The listing builds one solid part. Answer for the finished solid, in the listing's coordinates (mm). A direction names the side the tool comes from. Coordinates: 2 decimals unless noted, no trailing zeros. Loops run counter-clockwise (first coordinate to the right, second up) from the corner with the lowest first, then second, coordinate; pieces in that order, holes last. Notation, with made-up numbers: (81.5, -32.5) - (88.5, -32.5) arc R24 cw to (88.5, -8.5) - close; hole circle Ø2 at (-34.75, 22). An arc over 180 degrees is marked (long way). Write each question's results on one line, items separated by ' | '. Start each with the question number.
(1) Find section C-C on y = 24.5. Determine the outline of the cut face in (x, z) (3 decimals), then the cut area to 3 significant figures.
(2) Determine the mould class of faces 1 (the flat face through (-41, 50.165, 7)), 2 (the flat face through (1, 32, -7.938)), 3 (the flat face through (1, 35.052, -2)) for opening direction Y: released by +Y, released by -Y, zero draft, split by the parting line, or undercut.
(3) Find section B-B on x = 16. Determine the outline of the cut face in (y, z).
(4) For faces 4 (the flat face through (1, -35.052, -2)), 5 (the flat face through (-31.75, 52, 7)), 6 (the flat face through (-1, 45, 3.549)), determine the directions among +Z, -Z, +X, -X, +Y, -Y from which every point of the face is accessible in a straight line to the end or side of a thin tool.
(5) Find section A-A on z = -2.5. Determine the outline of the cut face in (x, y).
(6) Given pin 1 Ø5.5 at (x, z) = (-8.5, -3) entering from +Y; pin 2 Ø3.5 at (x, z) = (21.5, -2) entering from -Y; pin 3 Ø3 at (x, y) = (20.5, 33) entering from +Z, each flat-ended and moving along its own axis, determine where each tip first touches the part or whether it passes through.
(7) Consider line 1 (Y direction, x = 19.5, z = -0.5); line 2 (Y direction, x = -3.5, z = 4.25); line 3 (X direction, y = -45, z = 7) (3 decimals). Determine where each line is inside the solid, lowest interval first. Write a range as from..to.
(8) Find section D-D on y = -43. Determine the outline of the cut face in (x, z) (3 decimals).
from build123d import *

# Parameters (mm, degrees)
F1_DEPTH      = 54.7751
F1_DEPTH_BACK = 54.7751
F3_DEPTH      = 54.7761
F3_DEPTH_BACK = 54.7761
F4_W          = 109.5502
F4_H          = 5.9763903179
F5_DEPTH      = 54.7751
F5_DEPTH_BACK = 54.7751
F7_DEPTH      = 4.4523903179
F8_W          = 57.404
F8_H          = 17.4625
F9_DEPTH      = 50.165
F9_DEPTH_BACK = 50.165
F10_W         = 1.27
F10_H         = 0.635
F10_W_2       = 0.635
F10_H_2       = 1.27
F11_DEPTH     = 4.4523903179


with BuildPart() as f1:
    # F0 (on Right) → F1 (new body, two sides)
    with BuildSketch(Plane.YZ) as f1_sk:
        Polygon((35.052, 9.525), (-35.052, 9.525), (-35.052, -7.9375), (-28.702, -7.9375), (-28.702, 0), (28.702, 0), (28.702, -7.9375), (35.052, -7.9375), align=None)
    extrude(amount=F1_DEPTH)
    extrude(f1_sk.sketch, amount=-F1_DEPTH_BACK)

    # F2 (on Right) → F3 (cut, two sides)
    with BuildSketch(Plane.YZ) as f3_sk:
        with BuildLine():
            ThreePointArc((28.702, 0), (0, 3.5486096821), (-28.702, 0))
            Line((-28.702, 0), (28.702, 0))
        make_face()
    extrude(amount=F3_DEPTH, mode=Mode.SUBTRACT)
    extrude(f3_sk.sketch, amount=-F3_DEPTH_BACK, mode=Mode.SUBTRACT)

    # F4 (on Right) → F5 (join, two sides)
    with BuildSketch(Plane.YZ) as f5_sk:
        with Locations((0, 6.536804841)):
            Rectangle(F4_W, F4_H)
    extrude(amount=F5_DEPTH)
    extrude(f5_sk.sketch, amount=-F5_DEPTH_BACK)

    # F6 (on face) → F7 (cut, through all)
    with BuildSketch(Plane.XY.offset(9.525)):
        Polygon((50.165, -50.165), (50.165, 50.165), (31.75, 50.165), (31.75, 54.7751), (-31.75, 54.7751), (-31.75, 50.165), (-50.165, 50.165), (-50.165, -50.165), (-31.75, -50.165), (-31.75, -54.7751), (31.75, -54.7751), (31.75, -50.165), align=None)
    extrude(amount=-F7_DEPTH, mode=Mode.SUBTRACT)

    # F8 (on Right) → F9 (cut, two sides)
    with BuildSketch(Plane.YZ) as f9_sk:
        with Locations((0, 0.79375)):
            Rectangle(F8_W, F8_H)
    extrude(amount=F9_DEPTH, mode=Mode.SUBTRACT)
    extrude(f9_sk.sketch, amount=-F9_DEPTH_BACK, mode=Mode.SUBTRACT)

    # F10 (on face) → F11 (join, through all)
    with BuildSketch(Plane.XY.offset(5.0726096821)):
        with Locations((-32.385, 49.8475)):
            Rectangle(F10_W, F10_H)
        with Locations((32.385, 49.8475)):
            Rectangle(F10_W, F10_H)
        with Locations((-32.385, -49.8475)):
            Rectangle(F10_W, F10_H)
        with Locations((32.385, -49.8475)):
            Rectangle(F10_W, F10_H)
        with Locations((-49.8475, 0)):
            Rectangle(F10_W_2, F10_H_2)
        with Locations((49.8475, 0)):
            Rectangle(F10_W_2, F10_H_2)
    extrude(amount=F11_DEPTH)


solid = f1.part
Values:
1) outline: (-54.775, 0.974) - (-50.165, 0.974) - (-50.165, 9.525) - (-54.775, 9.525) - close; (50.165, 0.974) - (54.775, 0.974) - (54.775, 9.525) - (50.165, 9.525) - close | area: 78.8 mm²
2) face 1: undercut | face 2: zero draft | face 3: released by +Y
3) outline: (-54.78, 3.55) - (-35.05, 3.55) - (-35.05, -7.94) - (-28.7, -7.94) - (-28.7, 5.07) - (-54.78, 5.07) - close; (28.7, -7.94) - (35.05, -7.94) - (35.05, 3.55) - (54.78, 3.55) - (54.78, 5.07) - (28.7, 5.07) - close
4) face 4: -Z, +X, -X, -Y | face 5: +Z, +Y, -Y | face 6: -Z, +X, -X, +Y
5) outline: (-54.78, -35.05) - (54.78, -35.05) - (54.78, -28.7) - (-54.78, -28.7) - close; (-54.78, 28.7) - (54.78, 28.7) - (54.78, 35.05) - (-54.78, 35.05) - close
6) pin 1: stops at y = 35.05 | pin 2: stops at y = -35.05 | pin 3: stops at z = 5.07
7) line 1: y = -35.05..-28.7, 28.7..35.05 | line 2: y = -54.78..-28.7, 28.7..54.78 | line 3: x = -54.775..-50.165, 50.165..54.775
8) outline: (-54.775, 3.549) - (54.775, 3.549) - (54.775, 9.525) - (50.165, 9.525) - (50.165, 5.073) - (-50.165, 5.073) - (-50.165, 9.525) - (-54.775, 9.525) - close
